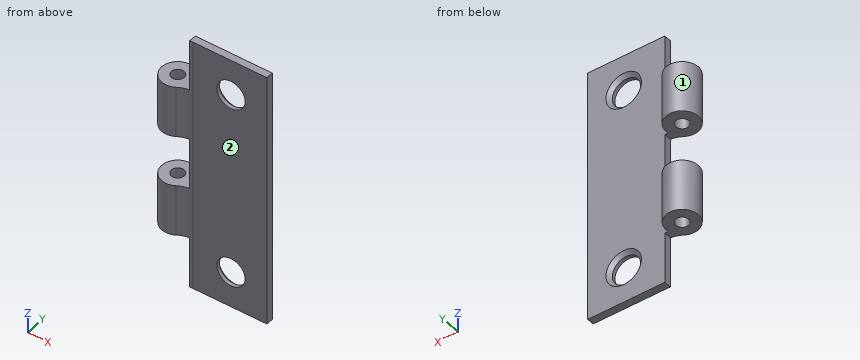
```python
from build123d import *

# Parameters (mm, degrees)
SKETCH4_R               = 3.175
BOSS_EXTRUDE2_DEPTH     = 25.4
FILLET1_R               = 5.08
M5_CLEARANCE_HOLE1_D    = 5.6
CUT_EXTRUDE1_DEPTH      = 32.908355123
CUT_EXTRUDE1_DEPTH_BACK = 32.908355123
SKETCH9_W               = 6.985
SKETCH9_H               = 10.16
SKETCH10_R              = 1.27
CUT_EXTRUDE2_DEPTH      = 55.347245805
CHAMFER1_SIZE           = 0.7112


with BuildPart() as part:
    # Sketch4 → Boss-Extrude2 (new, symmetric)
    with BuildSketch(Plane.XY):
        Circle(SKETCH4_R)
        with BuildLine():
            Line((19.050000043, -1.905), (19.050000043, -0.4826))
            Line((19.050000043, -0.4826), (3.138108067, -0.4826))
            ThreePointArc((3.138108067, -0.4826), (2.926778646, -1.230687513), (2.54, -1.905))
            Line((2.54, -1.905), (19.050000043, -1.905))
        make_face()
    extrude(amount=BOSS_EXTRUDE2_DEPTH, both=True)

    # Fillet1
    fillet1_edges = [part.edges().sort_by_distance(p)[0] for p in [
        (2.54, -1.905, 0),
    ]]
    fillet(fillet1_edges, radius=FILLET1_R)

    # M5 Clearance Hole1 (through all)
    with Locations(Plane(origin=(0, -0.4826, 0), x_dir=(1, 0, 0), z_dir=(0, 1, 0))):
        with Locations((11.938000043, 18.288), (11.938000043, -18.288)):
            Hole(M5_CLEARANCE_HOLE1_D / 2)

    # Sketch9 → Cut-Extrude1 (cut, two sides: drawn at the far end of the back side and taken through both)
    with BuildSketch(Plane(origin=(0, 0, 0), x_dir=(1, 0, 0), z_dir=(0, 1, 0)).offset(-CUT_EXTRUDE1_DEPTH_BACK)):
        with Locations((0.3175, -20.32)):
            Rectangle(SKETCH9_W, SKETCH9_H)
        with Locations((0.3175, 0)):
            Rectangle(SKETCH9_W, SKETCH9_H)
        with Locations((0.3175, 20.32)):
            Rectangle(SKETCH9_W, SKETCH9_H)
    extrude(amount=CUT_EXTRUDE1_DEPTH + CUT_EXTRUDE1_DEPTH_BACK, mode=Mode.SUBTRACT)

    # Sketch10 → Cut-Extrude2 (cut, through all)
    with BuildSketch(Plane.XY.offset(25.4)):
        Circle(SKETCH10_R)
    extrude(amount=-CUT_EXTRUDE2_DEPTH, mode=Mode.SUBTRACT)

    # Chamfer1
    chamfer1_edges = [part.edges().sort_by_distance(p)[0] for p in [
        (14.738000043, -0.4826, 18.288),
        (14.738000043, -0.4826, -18.288),
    ]]
    chamfer(chamfer1_edges, length=CHAMFER1_SIZE)


solid = part.part
```
Input: part model. Units: mm. Frame: model coordinates. Face numbers are marked on the shaded views. A direction names the side the tool comes from. Round coordinates to 2 decimals unless told otherwise and drop trailing zeros. Loops run counter-clockwise (first coordinate to the right, second up) from the corner with the lowest first, then second, coordinate; pieces in that order, holes last. Notation, with made-up numbers: (-17.5, -38.5) -> (28.5, -38.5) arc R22 ccw to (28.5, -1.5) -> close; hole circle Ø11 at (28.25, -18). An arc over 180 degrees is marked (long way). Use one line per item in the form item = value. Start each with the question number.
Item 1: Set-up query: the marked faces 1 and 2. Return all of +Z, -Z, +X, -X, +Y, -Y with unobstructed straight access to the full face (end or side cutting, diameter ignored); none if empty.
Item 2: Material intervals for L1, parallel to Z at x = -0.5, y = -1.25; L2, parallel to Y at x = 0, z = 10.75 (3 decimals); L3, parallel to Y at x = 16.5, z = -5 (3 decimals), sorted ascending. Write a range as from..to.
Item 3: Section query C-C on z = -11. Return the cut outline in (x, y) (3 decimals).
Item 4: Section query A-A on y = 0. Return the cut outline in (x, z) (3 decimals).
Item 5: Contact query for flat-ended pins moving along their axis: pin 1 Ø6.5 at (x, z) = (11.938, 18.288) entering from +Y; pin 2 Ø4 at (x, z) = (4, 13) entering from +Y; pin 3 Ø11.5 at (x, z) = (11.5, 7) entering from -Y (3 decimals). Output: stop coordinate, or through.
Item 6: Section query D-D on z = 0. Return the cut outline in (x, y) (3 decimals).
Ans:
q1.face_1 = +Z, -Z
q1.face_2 = +Z, -Z, +X, -Y
q2.L1 = -15.24..-5.08, 5.08..15.24
q2.L2 = -3.175..-1.27, 1.27..3.175
q2.L3 = -1.905..-0.483
q3.outline = (1.692, -2.687) arc R5.08 cw to (4.399, -1.905) -> (19.05, -1.905) -> (19.05, -0.483) -> (3.138, -0.483) arc R3.175 ccw (long way) to start; hole circle Ø2.54 at (0, 0)
q4.outline = (-3.175, -15.24) -> (-1.27, -15.24) -> (-1.27, -5.08) -> (-3.175, -5.08) -> close; (-3.175, 5.08) -> (-1.27, 5.08) -> (-1.27, 15.24) -> (-3.175, 15.24) -> close; (1.27, -15.24) -> (3.175, -15.24) -> (3.175, -5.08) -> (1.27, -5.08) -> close; (1.27, 5.08) -> (3.175, 5.08) -> (3.175, 15.24) -> (1.27, 15.24) -> close
q5.pin_1 = -0.74
q5.pin_2 = 2.47
q5.pin_3 = -1.905
q6.outline = (3.81, -1.939) arc R5.08 cw to (4.399, -1.905) -> (19.05, -1.905) -> (19.05, -0.483) -> (3.81, -0.483) -> close
